from build123d import *

# Parameters (mm, degrees)
SKETCH1_R           = 2.25
BOSS_EXTRUDE1_DEPTH = 6
SKETCH2_W           = 6.1
SKETCH2_H           = 6.1
BOSS_EXTRUDE2_DEPTH = 20
SKETCH3_W           = 5
SKETCH3_H           = 5
BOSS_EXTRUDE3_DEPTH = 8.7
SKETCH4_OUTSIDE_W   = 15.252
SKETCH4_OUTSIDE_H   = 15.252
SKETCH4_OUTSIDE_W_2 = 4.836378696
SKETCH4_OUTSIDE_H_2 = 4.876198926
CUT_EXTRUDE1_DEPTH  = 4
SKETCH5_W           = 3.5
SKETCH5_H           = 10
BOSS_EXTRUDE4_DEPTH = 2


with BuildPart() as part:
    # Sketch1 → Boss-Extrude1 (new body)
    with BuildSketch(Plane(origin=(0, 0, 0), x_dir=(1, 0, 0), z_dir=(0, 1, 0))):
        with Locations(Location((0, 0, 0), (0, 0, 270))):
            Circle(SKETCH1_R)
    extrude(amount=BOSS_EXTRUDE1_DEPTH)

    # Sketch2 → Boss-Extrude2 (add)
    with BuildSketch(Plane(origin=(0, 6, 0), x_dir=(1, 0, 0), z_dir=(0, 1, 0))):
        Rectangle(SKETCH2_W, SKETCH2_H)
    extrude(amount=BOSS_EXTRUDE2_DEPTH)

    # Sketch3 → Boss-Extrude3 (add)
    with BuildSketch(Plane(origin=(0, 26, 0), x_dir=(1, 0, 0), z_dir=(0, 1, 0))):
        Rectangle(SKETCH3_W, SKETCH3_H)
    extrude(amount=BOSS_EXTRUDE3_DEPTH)

    # Sketch4 outside → Cut-Extrude1 (cut)
    with BuildSketch(Plane(origin=(0, 34.7, 0), x_dir=(1, 0, 0), z_dir=(0, 1, 0))):
        Rectangle(SKETCH4_OUTSIDE_W, SKETCH4_OUTSIDE_H)
        Rectangle(SKETCH4_OUTSIDE_W_2, SKETCH4_OUTSIDE_H_2, mode=Mode.SUBTRACT)
    extrude(amount=-CUT_EXTRUDE1_DEPTH, mode=Mode.SUBTRACT)

    # Sketch5 → Boss-Extrude4 (add)
    with BuildSketch(Plane.XY.offset(3.05)):
        with Locations((0, 11)):
            Rectangle(SKETCH5_W, SKETCH5_H)
    extrude(amount=BOSS_EXTRUDE4_DEPTH)


solid = part.part
Work out the finished part from the listing and answer in its coordinate system (mm). A direction names the side the tool comes from. Coordinates: 2 decimals unless noted, no trailing zeros. Loops run counter-clockwise (first coordinate to the right, second up) from the corner with the lowest first, then second, coordinate; pieces in that order, holes last. Notation, with made-up numbers: M -24,60 L -5,60 A25 cw -5,94 Z; hole C 2,31.25 d9. An arc over 180 degrees is marked long. Answer in a Markdown table with one row per item. Add a question column.
1. Flat-ended cylindrical pins translate along their axes: P1, Ø1.6, axis at y = 10.5, z = 4, coming from the -X side; P2, Ø1.2, axis at y = 33.5, z = -1, coming from the +X side; P3, Ø1.4, axis at x = 0.5, y = 29, coming from the -Z side; P4, Ø1.8, axis at x = 0, z = 0, coming from the -Y side. Find the tip coordinate at first contact, or state that the pin passes through.
2. Find section C-C, the plane z = 0. Write down the section's boundary in (x, y).
3. Find section D-D, the plane y = 16.5. Write down the section's boundary in (x, z), then the cut area to 3 significant figures.
4. A tool of negligible diameter and unlimited length cuts with its end or side. For faces 1 (the flat face through (-2.418, 33, 0)), 2 (the flat face through (2.418, 33, 0)), 3 (the flat face through (0, 28, 2.5)), 4 (the cylindrical face through (0.676, 2.958, 2.146)), 5 (the flat face through (-1.75, 11, 4)), from which of +Z, -Z, +X, -X, +Y, -Y can it reach the whole face along a straight path? Write none if from no direction.
5. Consider L1, parallel to X at y = 8.5, z = 3.25; L2, parallel to X at y = 28, z = 0.5; L3, parallel to Y at x = -2, z = 1.5. Determine where each line is inside the solid, lowest interval first.
6. Find section B-B, the plane x = 0. Write down the section's boundary in (y, z), then the cut area to 3 significant figures.
7. Find section A-A, the plane y = 6.5. Write down the section's boundary in (x, z), then the cut area to 3 significant figures.
Reported:
| question | item | result |
|---|---|---|
| 1 | P1 | stops at x = -1.75 |
| 1 | P2 | stops at x = 2.42 |
| 1 | P3 | stops at z = -2.5 |
| 1 | P4 | stops at y = 0 |
| 2 | outline | M -3.05,6 L -2.25,6 L -2.25,0 L 2.25,0 L 2.25,6 L 3.05,6 L 3.05,26 L 2.5,26 L 2.5,30.7 L 2.42,30.7 L 2.42,34.7 L -2.42,34.7 L -2.42,30.7 L -2.5,30.7 L -2.5,26 L -3.05,26 Z |
| 3 | outline | M -3.05,-3.05 L 3.05,-3.05 L 3.05,3.05 L -3.05,3.05 Z |
| 3 | area | 37.2 mm^2 |
| 4 | face 1 | +Z, -Z, -X, +Y |
| 4 | face 2 | +Z, -Z, +X, +Y |
| 4 | face 3 | +Z, +X, -X, +Y |
| 4 | face 4 | -Y |
| 4 | face 5 | +Z, -X, +Y, -Y |
| 5 | L1 | x = -1.75 to 1.75 |
| 5 | L2 | x = -2.5 to 2.5 |
| 5 | L3 | y = 6 to 34.7 |
| 6 | outline | M 0,-2.25 L 6,-2.25 L 6,-3.05 L 26,-3.05 L 26,-2.5 L 30.7,-2.5 L 30.7,-2.44 L 34.7,-2.44 L 34.7,2.44 L 30.7,2.44 L 30.7,2.5 L 26,2.5 L 26,3.05 L 16,3.05 L 16,5.05 L 6,5.05 L 6,2.25 L 0,2.25 Z |
| 6 | area | 212 mm^2 |
| 7 | outline | M -3.05,-3.05 L 3.05,-3.05 L 3.05,3.05 L 1.75,3.05 L 1.75,5.05 L -1.75,5.05 L -1.75,3.05 L -3.05,3.05 Z |
| 7 | area | 44.2 mm^2 |
